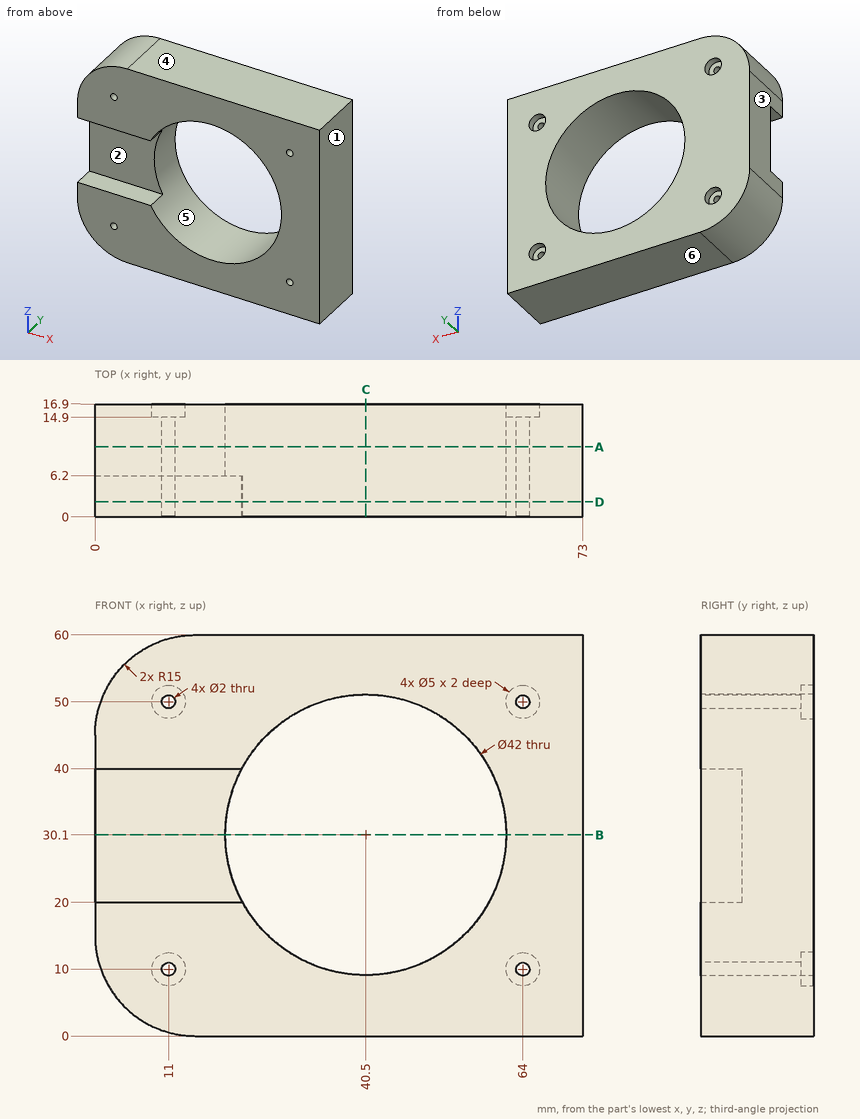
The figure shows three views and two pictorial views of one solid part (mm, origin at its lowest corner). Answer the questions. A direction names the side the tool comes from. Give positions to 0.01 mm unless a question says otherwise; leave off trailing zeros. Order: outer loops, then holes, each group sorted by start corner. A loop starts at its lowest first (then second) coordinate and runs counter-clockwise, first axis right, second up. Notation, with made-up numbers: (8.5, -31.5) -> (34.5, -31.5) arc R23 cw to (34.5, -14.5) -> close; hole circle Ø6 at (-29, 71.5). An arc over 180 degrees is marked (long way). Answer as CSV lines item,"result". Start each with the question number.
Q1. Which of the six approach directions +Z, -Z, +X, -X, +Y, -Y give full straight-line access (tool end or side, diameter ignored) to the marked faces 1 and 2?
Q2. Find the intervals of material crossed by L1, parallel to Z at x = 64, y = 4.5; L2, parallel to Z at x = 14.5, y = 1.75; L3, parallel to Z at x = 40.5, y = 8.5, in increasing order.
Q3. A cutting plane is placed at C-C (x = 40.5). Determine the outline of the cut face in (y, z).
Q4. A cutting plane is placed at A-A (y = 10.5). Determine the outline of the cut face in (x, z).
Q5. Determine the mould class of the marked faces 3, 4, 5 and 6 for opening direction Z: pulls with the +Z half, pulls with the -Z half, needs draft (parallel to the pull), parting line crosses it, or undercut.
Q6. A cutting plane is placed at D-D (y = 2.25). Determine the outline of the cut face in (x, z), then the cut area to 3 significant figures.
Q7. Given pin 1 (4 mm diameter, centred on x = 11, y = 7, fed in from +Z); pin 2 (8 mm diameter, centred on x = 11, z = 10, fed in from +Y); pin 3 (4 mm diameter, centred on x = 64, z = 50, fed in from +Y); pin 4 (3 mm diameter, centred on x = 7.5, y = 1.5, fed in from +Z), each flat-ended and moving along its own axis, determine where each tip first touches the part or whether it passes through.
Q8. A cutting plane is placed at B-B (z = 30.1). Determine the outline of the cut face in (x, y).
Results found:
1,face 1,"+Z, -Z, +X, +Y, -Y"
1,face 2,"-X, -Y"
2,L1,"0 to 9, 11 to 49, 51 to 60"
2,L2,"0.01 to 20, 40 to 59.99"
2,L3,"0 to 9.1, 51.1 to 60"
3,outline,"(0, 0) -> (16.9, 0) -> (16.9, 9.1) -> (0, 9.1) -> close; (0, 51.1) -> (16.9, 51.1) -> (16.9, 60) -> (0, 60) -> close"
4,outline,"(0, 15) arc R15 ccw to (15, 0) -> (73, 0) -> (73, 60) -> (15, 60) arc R15 ccw to (0, 45) -> close; hole circle Ø2 at (11, 10); hole circle Ø2 at (11, 50); hole circle Ø42 at (40.5, 30.1); hole circle Ø2 at (64, 10); hole circle Ø2 at (64, 50)"
5,face 3,"needs draft"
5,face 4,"pulls with the +Z half"
5,face 5,"undercut"
5,face 6,"pulls with the -Z half"
6,outline,"(0, 15) arc R15 ccw to (15, 0) -> (73, 0) -> (73, 60) -> (15, 60) arc R15 ccw to (0, 45) -> (0, 40) -> (21.98, 40) arc R21 cw (long way) to (22.09, 20) -> (0, 20) -> close; hole circle Ø2 at (11, 10); hole circle Ø2 at (11, 50); hole circle Ø2 at (64, 10); hole circle Ø2 at (64, 50)"
6,area,"2,480 mm2"
7,pin 1,"z = 59.87"
7,pin 2,"y = 16.9"
7,pin 3,"y = 14.9"
7,pin 4,"z = 58.75"
8,outline,"(0, 6.2) -> (19.5, 6.2) -> (19.5, 16.9) -> (0, 16.9) -> close; (61.5, 0) -> (73, 0) -> (73, 16.9) -> (61.5, 16.9) -> close"
